Source: CAD feature listing. Evaluate the final solid. Frame: model axes, mm. Face numbers are marked on the shaded views. A direction names the side the tool comes from. Coordinates: 2 decimals unless noted, no trailing zeros. Write each loop counter-clockwise with the first axis right and the second up, starting at its lowest first coordinate (ties: lowest second). Pieces come first, ordered by that corner, then holes. Notation, with made-up numbers: M 78,-28.75 L 124,-28.75 A31 ccw 124,7.25 Z; hole C 56.5,-16 d2. An arc over 180 degrees is marked long. One line per item, written item: value. Start each with the question number.
Item 1: Cut plane A-A, the plane x = 46. Output: boundary loops of the cut face in (y, z), then the cut area to 3 significant figures.
Item 2: Pin query (flat end, axial travel): P1, Ø8, axis at y = 67, z = -2, coming from the -X side; P2, Ø6.5, axis at x = 86, y = -45, coming from the -Z side; P3, Ø3.5, axis at y = 45, z = 23.5, coming from the +X side; P4, Ø10, axis at x = 112, z = -9.5, coming from the -Y side. Return the tip coordinate at first contact, or that it passes through.
Item 3: Mould query, pull axis Y, two halves, no side actions, for the marked faces 1, 2, 3 and 4. Classes: released by +Y, released by -Y, zero draft, split by the parting line, or undercut.
Item 4: Set-up query: the marked faces 5, 6 and 7. Return all of +Z, -Z, +X, -X, +Y, -Y with unobstructed straight access to the full face (end or side cutting, diameter ignored); none if empty.
Item 5: Ray query, L1, parallel to Z at x = 7.5, y = -5; L2, parallel to Z at x = 23, y = 68; L3, parallel to X at y = 15, z = -36.5. Return the intervals inside material, ascending. Write a range as from..to.
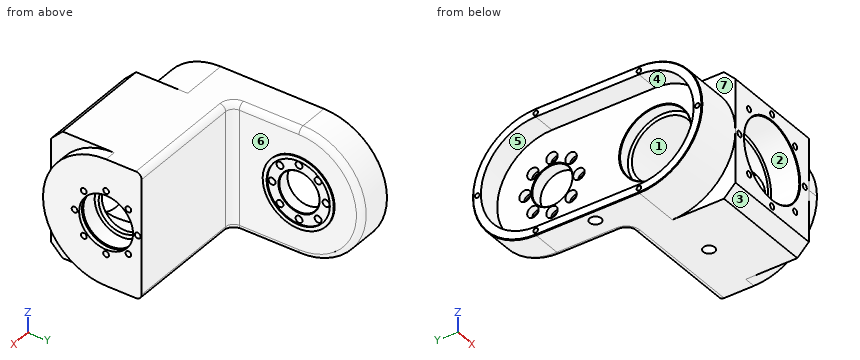
```python
from build123d import *

# Parameters (mm, degrees)
EXTRUDE_1_DEPTH                = 41
EXTRUDE_2_DEPTH                = 90
EXTRUDE_3_DEPTH                = 10
CUT_EXTRUDE_1_DEPTH            = 182.400110254
CUT_EXTRUDE_1_DEPTH_BACK       = 182.400110254
SKETCH_4_W                     = 10
SKETCH_4_H                     = 114
SKETCH_5_R                     = 31
SKETCH_5_R_2                   = 27.55
EXTRUDE_4_DEPTH                = 1
CUT_EXTRUDE_2_DEPTH            = 20
SKETCH_7_R                     = 2
CUT_EXTRUDE_3_DEPTH            = 12
CUT_EXTRUDE_4_REACH            = 206.893
SKETCH_8_R                     = 5
SKETCH_10_R                    = 17.5
CUT_EXTRUDE_5_DEPTH            = 167.330995308
PATTERN_CIRCULAR_1_COUNT       = 8
SKETCH_14_R                    = 2.5
CUT_EXTRUDE_6_DEPTH            = 15
SKETCH_15_R                    = 34
CUT_EXTRUDE_7_DEPTH            = 25
SKETCH_16_R                    = 30
CUT_EXTRUDE_8_DEPTH            = 25
SKETCH_17_R                    = 2.5
CUT_EXTRUDE_9_DEPTH            = 15
HOLE_WIZARD_M1_6_2_D           = 4
HOLE_WIZARD_M1_6_2_DEPTH       = 30
HOLE_WIZARD_M1_6_2_CBORE_D     = 10
HOLE_WIZARD_M1_6_2_CBORE_DEPTH = 12
HOLE_WIZARD_M1_6_2_TIP         = 1.201721238
FILLET_2_R                     = 7
FILLET_1_R                     = 5
CHAMFER_1_SIZE                 = 0.5


with BuildPart() as part:
    # 草图1 → 凸台-拉伸1 (new body)
    with BuildSketch(Plane(origin=(0, 0, 0), x_dir=(0, 0, -1), z_dir=(1, 0, 0))):
        with BuildLine():
            Line((55, 45), (55, -45))
            ThreePointArc((55, -45), (0, -100), (-55, -45))
            Line((-55, -45), (-55, 45))
            ThreePointArc((-55, 45), (0, 100), (55, 45))
        make_face()
    extrude(amount=EXTRUDE_1_DEPTH)

    # 草图2 → 凸台-拉伸2 (add)
    with BuildSketch(Plane(origin=(41, 0, 0), x_dir=(0, 0, -1), z_dir=(1, 0, 0))):
        Polygon((-55, -14), (55, -14), (55, -90), (45, -100), (-45, -100), (-55, -90), align=None)
    extrude(amount=EXTRUDE_2_DEPTH)

    # 草图3 → 凸台-拉伸3 (add)
    with BuildSketch(Plane(origin=(131, 0, 0), x_dir=(0, 0, -1), z_dir=(1, 0, 0))):
        with BuildLine():
            Line((55, -14), (-55, -14))
            Line((-55, -14), (-55, -45))
            ThreePointArc((-55, -45), (-38.890872965, -83.890872965), (0, -100))
            ThreePointArc((0, -100), (38.890872965, -83.890872965), (55, -45))
            Line((55, -45), (55, -14))
        make_face()
    extrude(amount=EXTRUDE_3_DEPTH)

    # 草图4 → 切除-拉伸1 (cut, two sides: drawn at the far end of the back side and taken through both)
    with BuildSketch(Plane.XY.offset(-CUT_EXTRUDE_1_DEPTH_BACK)):
        with Locations((36, 43)):
            Rectangle(SKETCH_4_W, SKETCH_4_H)
    extrude(amount=CUT_EXTRUDE_1_DEPTH + CUT_EXTRUDE_1_DEPTH_BACK, mode=Mode.SUBTRACT)

    # 草图5 → 凸台-拉伸4 (add)
    with BuildSketch(Plane(origin=(31, 0, 0), x_dir=(0, 0, -1), z_dir=(1, 0, 0))):
        with Locations(Location((0, 45, 0), (0, 0, 180))):
            Circle(SKETCH_5_R)
        with Locations((0, 45)):
            Circle(SKETCH_5_R_2, mode=Mode.SUBTRACT)
    extrude(amount=EXTRUDE_4_DEPTH)

    # 草图6 → 切除-拉伸2 (cut)
    with BuildSketch(Plane.ZY):
        with BuildLine():
            Line((47.75, 45), (47.75, -45))
            ThreePointArc((47.75, -45), (0, -92.75), (-47.75, -45))
            Line((-47.75, -45), (-47.75, 45))
            ThreePointArc((-47.75, 45), (0, 92.75), (47.75, 45))
        make_face()
    extrude(amount=-CUT_EXTRUDE_2_DEPTH, mode=Mode.SUBTRACT)

    # 草图7 → 切除-拉伸3 (cut)
    with BuildSketch(Plane.ZY):
        with Locations((0, 96)):
            Circle(SKETCH_7_R)
        with Locations((-51, 45)):
            Circle(SKETCH_7_R)
        with Locations((51, 45)):
            Circle(SKETCH_7_R)
        with Locations(Location((51, -45, 0), (0, 0, 180))):
            Circle(SKETCH_7_R)
        with Locations(Location((-51, -45, 0), (0, 0, 180))):
            Circle(SKETCH_7_R)
        with Locations(Location((0, -96, 0), (0, 0, 180))):
            Circle(SKETCH_7_R)
    extrude(amount=-CUT_EXTRUDE_3_DEPTH, mode=Mode.SUBTRACT)

    # 草图8 → 切除-拉伸4 (cut, up to next)
    with BuildSketch(Plane(origin=(0, 0, -55), x_dir=(-1, 0, 0), z_dir=(0, 0, -1)), mode=Mode.PRIVATE) as cut_extrude_4_sk1:
        with Locations((-10, 0)):
            Circle(SKETCH_8_R)
    cut_extrude_4_tool1 = extrude(cut_extrude_4_sk1.sketch, amount=-CUT_EXTRUDE_4_REACH, mode=Mode.PRIVATE) & part.part
    add(cut_extrude_4_tool1.solids().sort_by_distance((10, 0, -55))[0], mode=Mode.SUBTRACT)

    # 草图10 → 切除-拉伸5 (cut, through all)
    with BuildSketch(Plane.ZY.offset(-20)):
        with Locations((0, 45)):
            Circle(SKETCH_10_R)
    extrude(amount=-CUT_EXTRUDE_5_DEPTH, mode=Mode.SUBTRACT)

    # 草图12 → M1.6 六角头螺栓的柱形沉头孔1 (revolve, cut)
    with BuildSketch(Plane(origin=(20, 68.5, 0), x_dir=(0, 0, 1), z_dir=(0, 1, 0))):
        Polygon((0, 0), (0, 16.802581857), (3, 15), (3, 6), (5, 6), (5, 0), align=None)
    hole_wizard_m1_6_1 = revolve(axis=Axis((13.65, 68.5, 0), (1, 0, 0)), mode=Mode.SUBTRACT)

    # 阵列(圆周)1: M1.6 六角头螺栓的柱形沉头孔1 ×8 about axis
    pattern_circular_1_axis = Axis((0, 45, 0), (1, 0, 0))
    for i in range(1, PATTERN_CIRCULAR_1_COUNT):
        add(hole_wizard_m1_6_1.rotate(pattern_circular_1_axis, i * 360 / PATTERN_CIRCULAR_1_COUNT), mode=Mode.SUBTRACT)

    # 草图13 → 切除-旋转1 (revolve, cut)
    with BuildSketch(Plane.XY, mode=Mode.PRIVATE) as cut_revolve_1_sk:
        Polygon((20, -45), (20, -14), (30, -14), (30, -17.5), (118, -17.5), (118, -25), (122, -25), (122, -21.5), (136, -21.5), (136, -20.5), (137.5, -20.5), (137.5, -21.5), (141, -21.5), (141, -45), align=None)
    revolve(cut_revolve_1_sk.sketch.rotate(Axis((20, -45, 0), (1, 0, 0)), 180), axis=Axis((20, -45, 0), (1, 0, 0)), mode=Mode.SUBTRACT)

    # 草图14 → 切除-拉伸6 (cut)
    with BuildSketch(Plane(origin=(141, 0, 0), x_dir=(0, 0, -1), z_dir=(1, 0, 0))):
        with Locations((0, -17.5)):
            Circle(SKETCH_14_R)
        with Locations((19.445436483, -25.554563517)):
            Circle(SKETCH_14_R)
        with Locations((27.5, -45)):
            Circle(SKETCH_14_R)
        with Locations((19.445436483, -64.445436483)):
            Circle(SKETCH_14_R)
        with Locations((0, -72.5)):
            Circle(SKETCH_14_R)
        with Locations((-19.445436483, -64.445436483)):
            Circle(SKETCH_14_R)
        with Locations((-27.5, -45)):
            Circle(SKETCH_14_R)
        with Locations((-19.445436483, -25.554563517)):
            Circle(SKETCH_14_R)
    extrude(amount=-CUT_EXTRUDE_6_DEPTH, mode=Mode.SUBTRACT)

    # 草图15 → 切除-拉伸7 (cut)
    with BuildSketch(Plane.XZ.offset(100)):
        with Locations(Location((86, 0, 0), (0, 0, 270))):
            Circle(SKETCH_15_R)
    extrude(amount=-CUT_EXTRUDE_7_DEPTH, mode=Mode.SUBTRACT)

    # 草图16 → 切除-拉伸8 (cut)
    with BuildSketch(Plane.XZ.offset(75)):
        with Locations(Location((86, 0, 0), (0, 0, 270))):
            Circle(SKETCH_16_R)
    extrude(amount=-CUT_EXTRUDE_8_DEPTH, mode=Mode.SUBTRACT)

    # 草图17 → 切除-拉伸9 (cut)
    with BuildSketch(Plane.XZ.offset(100)):
        with Locations(Location((86, 40, 0), (0, 0, 270))):
            Circle(SKETCH_17_R)
        with Locations(Location((114.284271247, 28.284271247, 0), (0, 0, 270))):
            Circle(SKETCH_17_R)
        with Locations(Location((126, 0, 0), (0, 0, 270))):
            Circle(SKETCH_17_R)
        with Locations(Location((114.284271247, -28.284271247, 0), (0, 0, 270))):
            Circle(SKETCH_17_R)
        with Locations(Location((86, -40, 0), (0, 0, 270))):
            Circle(SKETCH_17_R)
        with Locations(Location((57.715728753, -28.284271247, 0), (0, 0, 270))):
            Circle(SKETCH_17_R)
        with Locations(Location((46, 0, 0), (0, 0, 270))):
            Circle(SKETCH_17_R)
        with Locations(Location((57.715728753, 28.284271247, 0), (0, 0, 270))):
            Circle(SKETCH_17_R)
    extrude(amount=-CUT_EXTRUDE_9_DEPTH, mode=Mode.SUBTRACT)

    # M1.6 六角头螺栓的柱形沉头孔2
    with Locations(Plane(origin=(0, 0, -55), x_dir=(-1, 0, 0), z_dir=(0, 0, -1))):
        with Locations((-86, -45)):
            CounterBoreHole(HOLE_WIZARD_M1_6_2_D / 2, HOLE_WIZARD_M1_6_2_CBORE_D / 2, HOLE_WIZARD_M1_6_2_CBORE_DEPTH, depth=HOLE_WIZARD_M1_6_2_DEPTH)
            with Locations((0, 0, -(HOLE_WIZARD_M1_6_2_DEPTH + HOLE_WIZARD_M1_6_2_TIP / 2))):  # 118° drill point
                Cone(0, HOLE_WIZARD_M1_6_2_D / 2, HOLE_WIZARD_M1_6_2_TIP, mode=Mode.SUBTRACT)

    # 圆角2
    fillet_2_edges = [part.edges().sort_by_distance(p)[0] for p in [
        (31, -14, 0),
    ]]
    fillet(fillet_2_edges, radius=FILLET_2_R)

    # 圆角1
    fillet_1_edges = [part.edges().sort_by_distance(p)[0] for p in [
        (89.5, -14, 55),
        (89.5, -14, -55),
        (33.050252532, -11.949747468, 55),
        (33.050252532, -11.949747468, -55),
        (31, 100, 0),
        (31, 19, -55),
        (31, 19, 55),
    ]]
    fillet(fillet_1_edges, radius=FILLET_1_R)

    # 倒角1
    chamfer_1_edges = [part.edges().sort_by_distance(p)[0] for p in [
        (31, 45, -17.5),
        (20, 45, -17.5),
        (20, -14, 0),
        (86, -100, 34),
        (0, 0, -55),
        (0, -100, 0),
        (0, 0, 55),
        (0, 100, 0),
    ]]
    chamfer(chamfer_1_edges, length=CHAMFER_1_SIZE)


solid = part.part
```
From the geometry:
1. outline: M -100,-45 L -90,-55 L -19,-55 A5 ccw -14,-50 L -14,50 A5 ccw -19,55 L -90,55 L -100,45 L -100,2.5 L -85,2.5 L -85,-2.5 L -100,-2.5 Z; hole C -45,0 d55
1. area: 6,900 mm²
2. P1: stops at x = 20
2. P2: stops at z = -43
2. P3: passes through
2. P4: stops at y = -75
3. face 1: undercut
3. face 2: zero draft
3. face 3: released by -Y
3. face 4: undercut
4. face 5: -X
4. face 6: +X
4. face 7: +Z, -X, -Y
5. L1: z = -55..-47.75, 47.75..55
5. L2: z = -49.96..-4.97, 4.97..49.96
5. L3: x = 20..31
